```python
from build123d import *

# Parameters (mm, degrees)
F2_W     = 88.9
F2_H     = 15.875
F3_DEPTH = 31.75
F4_SIZE  = 6.35
F5_R     = 18.161
F6_DEPTH = 66.676
F7_SIZE  = 1.27


with BuildPart() as f1:
    # F0 (on Front) → F1 (revolve)
    with BuildSketch(Plane.XZ):
        with BuildLine():
            Line((-317.5, 0), (0, 0))
            Line((0, 0), (0, 19.05))
            ThreePointArc((0, 19.05), (-5.231581, 26.09159), (-11.935, 31.75))
            Line((-11.935, 31.75), (-298.45, 31.75))
            Line((-298.45, 31.75), (-298.45, 50.8))
            Line((-298.45, 50.8), (-317.5, 50.8))
            Line((-317.5, 50.8), (-317.5, 0))
        make_face()
    revolve(axis=Axis((-156.483173, 0, 0), (-1, 0, 0)))

    # F2 (on Top) → F3 (cut, symmetric)
    with BuildSketch(Plane.XY):
        with Locations((-44.45, 23.8125)):
            Rectangle(F2_W, F2_H)
        with Locations((-44.45, -23.8125)):
            Rectangle(F2_W, F2_H)
    extrude(amount=F3_DEPTH, both=True, mode=Mode.SUBTRACT)

    # F4
    f4_edges = [f1.edges().sort_by_distance(p)[0] for p in [
        (-88.9, -15.875, 0),
        (-88.9, 15.875, 0),
    ]]
    chamfer(f4_edges, length=F4_SIZE)

    # F5 (on face) → F6 (cut, through all)
    with BuildSketch(Plane.XZ.offset(15.875)):
        with Locations((-31.75, 0)):
            Circle(F5_R)
    extrude(amount=-F6_DEPTH, mode=Mode.SUBTRACT)

    # F7
    f7_edges = [f1.edges().sort_by_distance(p)[0] for p in [
        (-298.45, 0, -50.8),
        (-317.5, 0, -50.8),
    ]]
    chamfer(f7_edges, length=F7_SIZE)


solid = f1.part
```
Can you work these out from the model? Positions are in its coordinate system, mm. A direction names the side the tool comes from. Coordinates: 2 decimals unless noted, no trailing zeros. Loops run counter-clockwise (first coordinate to the right, second up) from the corner with the lowest first, then second, coordinate; pieces in that order, holes last.
1) Thinking about a two-plate mould opening in X: for faces 1 (the cylindrical face through (-45.14, -0.22, 12.27)), 2 (the flat face through (-85.769, 19.094, -0.385)), 3 (the cylindrical face through (-189.03, -12.16, 29.33)), which applies, pulls with the +X half, pulls with the -X half, needs draft (parallel to the pull), parting line crosses it, or undercut?
2) For pin 1 (10.5 mm diameter, centred on y = -28, z = -8, fed in from +X); pin 2 (10 mm diameter, centred on y = -1.5, z = 13, fed in from +X); pin 3 (2 mm diameter, centred on x = -171.5, y = -11.5, fed in from -Z); pin 4 (1.5 mm diameter, centred on x = -184, y = 26, fed in from -Z), each with a flat end and sliding along its axis, tell me the tip position at first contact or that it passes through.
3) Which directions (+Z, -Z, +X, -X, +Y, -Y) give clear straight access to the entire face, cutting with the end or side of a thin tool? Please do faces 4 (the flat face through (-51, -15.875, 0)), 5 (the flat face through (-51, 15.875, 0)), 6 (the flat face through (-298.45, -32, 1)), 7 (the flat face through (-317.5, 1, -1)).
4) Imagine slicing it at A-A on x = -31.75. List the corners of the cut face in (y, z) for me (3 decimals).
5) Imagine slicing it at C-C on x = -267. List the corners of the cut face in (y, z) for me, plus the area to 3 significant figures.
6) Imagine slicing it at B-B on z = 0. List the corners of the cut face in (x, y) for me (3 decimals).
7) I need wall thicknesses on probe 1 along Z at (x, y) = (-127, -26); probe 2 along Z at (x, y) = (-31.75, 8); probe 3 along X at (y, z) = (30, 5.5). Which ranges of each line are inside material? Lowest first, please.
Completed:
1. face 1: undercut
1. face 2: pulls with the +X half
1. face 3: needs draft
2. pin 1: stops at x = -88.9
2. pin 2: stops at x = 0
2. pin 3: stops at z = -29.96
2. pin 4: stops at z = -19.25
3. face 4: +Z, -Z, +X, -Y
3. face 5: +Z, -Z, +X, +Y
3. face 6: +X
3. face 7: +Z, -Z, -X, +Y, -Y
4. outline: (-15.875, -27.496) arc R31.75 ccw to (15.875, -27.496) - (15.875, -18.161) - (-15.875, -18.161) - close; (-15.875, 18.161) - (15.875, 18.161) - (15.875, 27.496) arc R31.75 ccw to (-15.875, 27.496) - close
5. outline: circle Ø63.5 at (0, 0)
5. area: 3,170 mm2
6. outline: (-317.5, -49.53) - (-316.23, -50.8) - (-299.72, -50.8) - (-298.45, -49.53) - (-298.45, -31.75) - (-88.9, -31.75) - (-88.9, -22.225) - (-82.55, -15.875) - (-49.911, -15.875) - (-49.911, 15.875) - (-82.55, 15.875) - (-88.9, 22.225) - (-88.9, 31.75) - (-298.45, 31.75) - (-298.45, 49.53) - (-299.72, 50.8) - (-316.23, 50.8) - (-317.5, 49.53) - close; (-13.589, -15.875) - (0, -15.875) - (0, 15.875) - (-13.589, 15.875) - close
7. probe 1: z = -18.22 to 18.22
7. probe 2: z = -30.73 to -18.16, 18.16 to 30.73
7. probe 3: x = -317.5 to -88.9
